```python
from build123d import *

# Parameters (mm, degrees)
SKETCH1_W           = 63.5
SKETCH1_H           = 50.8
BOSS_EXTRUDE1_DEPTH = 6.35
BOSS_EXTRUDE2_DEPTH = 15.875
FILLET1_R           = 12.7
FILLET2_R           = 6.35
BOSS_EXTRUDE5_DEPTH = 3.175
SKETCH5_R           = 2.413
CUT_EXTRUDE3_DEPTH  = 47.925927366
SKETCH8_R           = 2.25
CUT_EXTRUDE4_DEPTH  = 7.35


with BuildPart() as part:
    # Sketch1 → Boss-Extrude1 (new body)
    with BuildSketch(Plane(origin=(0, 0, 0), x_dir=(1, 0, 0), z_dir=(0, 1, 0))):
        Rectangle(SKETCH1_W, SKETCH1_H)
    extrude(amount=BOSS_EXTRUDE1_DEPTH)

    # Sketch2 → Boss-Extrude2 (add, symmetric)
    with BuildSketch(Plane.XY):
        Polygon((-11.43, 0), (13.036574415, 67.221360736), (7.069526273, 69.393188646), (-17.397048142, 2.17182791), align=None)
    extrude(amount=BOSS_EXTRUDE2_DEPTH, both=True)

    # Fillet1
    fillet1_edges = [part.edges().sort_by_distance(p)[0] for p in [
        (10.053050344, 68.307274691, 15.875),
        (10.053050344, 68.307274691, -15.875),
    ]]
    fillet(fillet1_edges, radius=FILLET1_R)

    # Fillet2
    fillet2_edges = [part.edges().sort_by_distance(p)[0] for p in [
        (-15.876317868, 6.35, 0),
        (-9.118789012, 6.35, 0),
    ]]
    fillet(fillet2_edges, radius=FILLET2_R)

    # Sketch7 → Boss-Extrude5 (add, symmetric)
    with BuildSketch(Plane.XY):
        with BuildLine():
            Line((4.748476913, 44.45), (31.75, 6.35))
            Line((31.75, 6.35), (-0.05004917, 6.35))
            ThreePointArc((-0.05004917, 6.35), (-5.251664651, 9.057789629), (-6.017097312, 14.87182791))
            Line((-6.017097312, 14.87182791), (4.748476913, 44.45))
        make_face()
        with BuildLine():
            Line((-31.75, 6.35), (-20.322635735, 6.35))
            ThreePointArc((-20.322635735, 6.35), (-16.680425364, 7.498384519), (-14.355587593, 10.52817209))
            Line((-14.355587593, 10.52817209), (-4.32026293, 38.1))
            Line((-4.32026293, 38.1), (-31.75, 6.35))
        make_face()
    extrude(amount=BOSS_EXTRUDE5_DEPTH, both=True)

    # Sketch5 → Cut-Extrude3 (cut, through all)
    with BuildSketch(Plane(origin=(-16.059992134, 5.845359099, 0), x_dir=(0, 0, 1), z_dir=(-0.939692621, 0.342020143, 0))):
        with Locations((0, 54.926187693)):
            Circle(SKETCH5_R)
    extrude(amount=-CUT_EXTRUDE3_DEPTH, mode=Mode.SUBTRACT)

    # Sketch8 → Cut-Extrude4 (cut, through all)
    with BuildSketch(Plane(origin=(0, 6.35, 0), x_dir=(1, 0, 0), z_dir=(0, 1, 0))):
        with Locations((10, -19.85)):
            Circle(SKETCH8_R)
        with Locations((10, 19.85)):
            Circle(SKETCH8_R)
        with Locations((-10, 19.85)):
            Circle(SKETCH8_R)
        with Locations((-10, -19.85)):
            Circle(SKETCH8_R)
    extrude(amount=-CUT_EXTRUDE4_DEPTH, mode=Mode.SUBTRACT)


solid = part.part
```
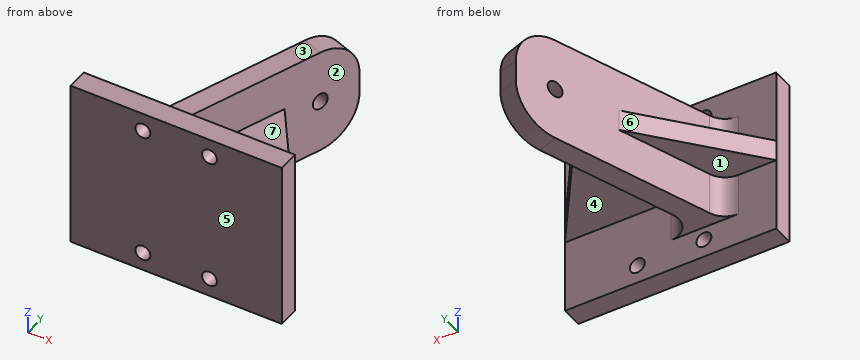
CAD build for the part. Positions are in the model's coordinates, mm. Face numbers are marked on the shaded views. A direction names the side the tool comes from. Round coordinates to 2 decimals unless told otherwise and drop trailing zeros. Write each loop counter-clockwise with the first axis right and the second up, starting at its lowest first coordinate (ties: lowest second). Pieces come first, ordered by that corner, then holes. Notation, with made-up numbers: (-36.5, -39) - (-24.5, -39) arc R22 ccw to (-24.5, -25) - close; hole circle Ø6 at (85, 89.25). An arc over 180 degrees is marked (long way). Write item = value, one per line. Start each with the question number.
Q1. Mould opens along Y. For the marked faces 5, 6 and 7 say: pulls with the +Y half, pulls with the -Y half, needs draft (parallel to the pull), parting line crosses it, or undercut.
Q2. Which spindle directions (+Z, -Z, +X, -X, +Y, -Y) get a long thin tool onto all of the face, cutting with end or side? Do the marked faces 1, 2, 3 and 4. Say none if no direction does.
Q3. Band-saw the part on D-D (y = 34.5). Give the cut face in (x, z) (3 decimals).
Q4. Band-saw the part on B-B (x = -10). Give the cut face in (y, z) (3 decimals), then the cut area to 3 significant figures.
Q5. Band-saw the part on A-A (z = 19.85). Give the cut face in (x, y).
Q6. Band-saw the part on C-C (z = 1). Give the cut face in (x, y), then the cut area to 3 significant figures.
Q7. Drop flat-ended pins along their axis: pin 1 (19 mm diameter, centred on x = 21, y = 25, fed in from +Z) (3 decimals); pin 2 (3 mm diameter, centred on x = 20, y = 20, fed in from -Z) (3 decimals); pin 3 (5 mm diameter, centred on x = -4, y = 27, fed in from -Z) (3 decimals); pin 4 (4 mm diameter, centred on x = 10, z = -19.85, fed in from +Y). Give the stop position or say it passes through.
Q8. Probe L1, parallel to Z at x = 10, y = 3.25; L2, parallel to X at y = 3, z = 19.85; L3, parallel to X at y = 1, z = -19. List the from-to ranges inside material, lowest first. Write a range as from..to.
Answers below:
q1.face_5 = pulls with the -Y half
q1.face_6 = pulls with the +Y half
q1.face_7 = undercut
q2.face_1 = -Z, -X, +Y
q2.face_2 = +X
q2.face_3 = +Z, +X, -X, +Y
q2.face_4 = -Z, +X
q3.outline = (-7.43, -3.175) - (-5.631, -3.175) - (-5.631, -15.875) - (1.127, -15.875) - (1.127, -3.175) - (11.8, -3.175) - (11.8, 3.175) - (1.127, 3.175) - (1.127, 15.875) - (-5.631, 15.875) - (-5.631, 3.175) - (-7.43, 3.175) - close
q4.outline = (0, -25.4) - (6.35, -25.4) - (6.35, -22.1) - (0, -22.1) - close; (0, -17.6) - (6.35, -17.6) - (6.35, -15.875) - (22.495, -15.875) - (22.495, -3.175) - (31.526, -3.175) - (31.526, 3.175) - (22.495, 3.175) - (22.495, 15.875) - (6.35, 15.875) - (6.35, 17.6) - (0, 17.6) - close; (0, 22.1) - (6.35, 22.1) - (6.35, 25.4) - (0, 25.4) - close
q4.area = 835 mm2
q5.outline = (-31.75, 0) - (-12.25, 0) - (-12.25, 6.35) - (-31.75, 6.35) - close; (-7.75, 0) - (7.75, 0) - (7.75, 6.35) - (-7.75, 6.35) - close; (12.25, 0) - (31.75, 0) - (31.75, 6.35) - (12.25, 6.35) - close
q6.outline = (-31.75, 0) - (31.75, 0) - (31.75, 6.35) - (4.75, 44.45) - (7.94, 53.22) - (1.97, 55.4) - (-4.32, 38.1) - (-31.75, 6.35) - close; (3.48, 59.52) - (9.44, 57.35) - (13.04, 67.22) - (7.07, 69.39) - close
q6.area = 1,820 mm2
q7.pin_1 = 3.175
q7.pin_2 = -3.175
q7.pin_3 = -15.875
q7.pin_4 = through
q8.L1 = -25.4..-22.1, -17.6..17.6, 22.1..25.4
q8.L2 = -31.75..-12.25, -7.75..7.75, 12.25..31.75
q8.L3 = -31.75..-12.08, -7.92..7.92, 12.08..31.75
